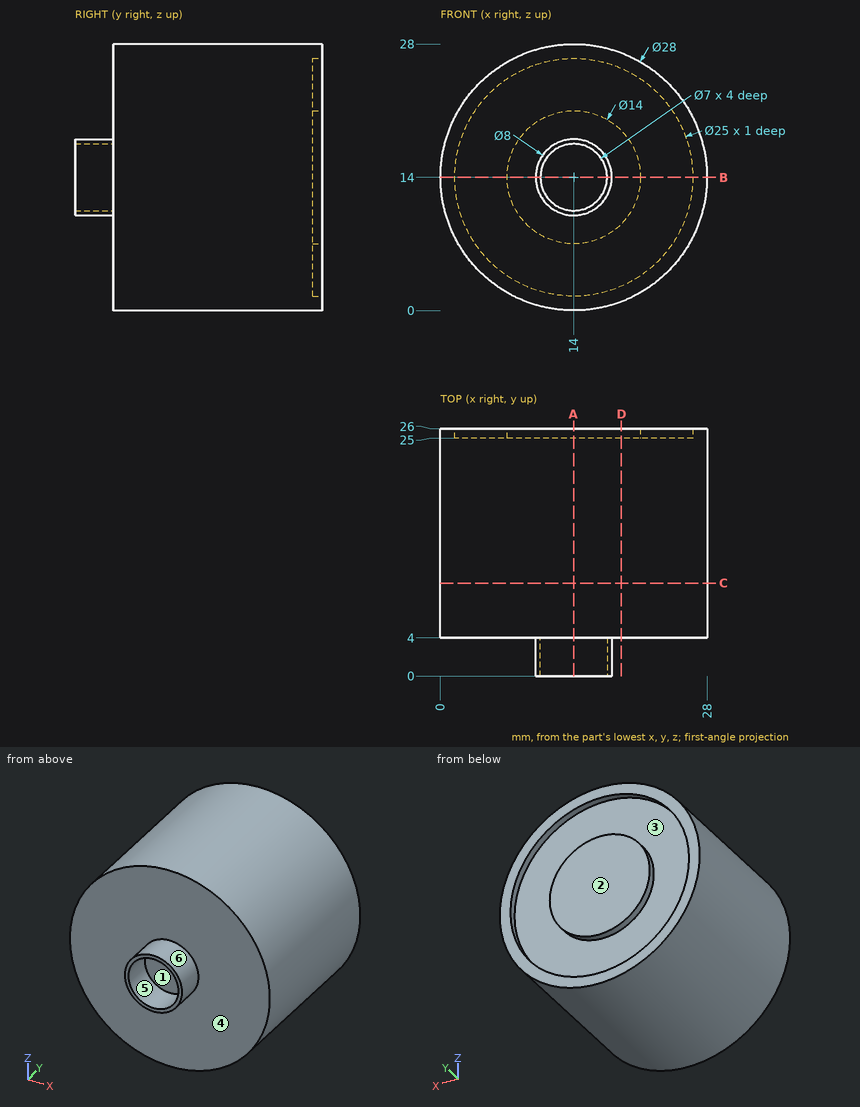
Design review of the part shown in the three views and the two pictorial views. Dimensions are in mm from the part's minimum x, y and z. A direction names the side the tool comes from. Coordinates: 2 decimals unless noted, no trailing zeros. Order: outer loops, then holes, each group sorted by start corner. A loop starts at its lowest first (then second) coordinate and runs counter-clockwise, first axis right, second up.
Item 1: For line 1 (Z direction, x = 14, y = 25.65); line 2 (Z direction, x = 14, y = 2.45); line 3 (Y direction, x = 11.5, z = 21.5), list the stretches that pass through material, from the lowest coordinate up.
Item 2: Take a section at D-D, the plane x = 19. Write out the cut boundary in (y, z), then the cut area to 3 significant figures.
Item 3: Take a section at A-A, the plane x = 14. Write out the cut boundary in (y, z), then the cut area to 3 significant figures.
Item 4: For the marked faces 1, 2 and 3, list the 3-axis set-ups (+Z, -Z, +X, -X, +Y, -Y) from which the entire face can be reached by the end or side of a thin tool; tool diameter is ignored.
Item 5: For pin 1 Ø8 at (x, y) = (19.5, 4) entering from -Z; pin 2 Ø2 at (y, z) = (22, 9) entering from +X; pin 3 Ø1.5 at (x, y) = (19, 7.5) entering from -Z, all flat-tipped, find the tip position at first contact; note any pin that passes through.
Item 6: Take a section at B-B, the plane z = 14. Write out the cut boundary in (x, y), then the cut area to 3 significant figures.
Item 7: Take a section at C-C, the plane y = 9.75. Write out the cut boundary in (x, z), then the cut area to 3 significant figures.
Item 8: The part is to be moulded in two halves that separate along Z. For the marked faces 4, 5 and 6, say which applies: pulls with the +Z half, pulls with the -Z half, needs draft (parallel to the pull), parting line crosses it, or undercut.
The answers:
1. line 1: z = 0 to 1.5, 7 to 21, 26.5 to 28
1. line 2: z = 10 to 10.5, 17.5 to 18
1. line 3: y = 4 to 25
2. outline: (4, 0.92) - (26, 0.92) - (26, 2.54) - (25, 2.54) - (25, 9.1) - (26, 9.1) - (26, 18.9) - (25, 18.9) - (25, 25.46) - (26, 25.46) - (26, 27.08) - (4, 27.08) - close
2. area: 562 mm2
3. outline: (0, 10) - (4, 10) - (4, 0) - (26, 0) - (26, 1.5) - (25, 1.5) - (25, 7) - (26, 7) - (26, 21) - (25, 21) - (25, 26.5) - (26, 26.5) - (26, 28) - (4, 28) - (4, 18) - (0, 18) - (0, 17.5) - (4, 17.5) - (4, 10.5) - (0, 10.5) - close
3. area: 609 mm2
4. face 1: -Y
4. face 2: +Z, -Z, +X, -X, +Y
4. face 3: +Y
5. pin 1: stops at z = 0.08
5. pin 2: stops at x = 27.42
5. pin 3: stops at z = 0.66
6. outline: (0, 4) - (10, 4) - (10, 0) - (10.5, 0) - (10.5, 4) - (17.5, 4) - (17.5, 0) - (18, 0) - (18, 4) - (28, 4) - (28, 26) - (26.5, 26) - (26.5, 25) - (21, 25) - (21, 26) - (7, 26) - (7, 25) - (1.5, 25) - (1.5, 26) - (0, 26) - close
6. area: 609 mm2
7. outline: circle Ø28 at (14, 14)
7. area: 616 mm2
8. face 4: needs draft
8. face 5: undercut
8. face 6: parting line crosses it
